from build123d import *
from build123d.topology import SkipClean

# Parameters (mm, degrees)
SKETCH_1_W           = 80
SKETCH_1_H           = 120
SKETCH_1_R           = 1.5
EXTRUDE_2_DEPTH      = 4
SKETCH_4_W           = 4
SKETCH_4_H           = 10
EXTRUDE_4_DEPTH      = 20
EXTRUDE_5_DEPTH      = 15
EXTRUDE_5_DEPTH_BACK = 10
SKETCH_5_W           = 20
SKETCH_5_H           = 4
CUT_EXTRUDE_1_REACH  = 132.959
SKETCH_6_R           = 1.6
CUT_EXTRUDE_START    = -50
CUT_EXTRUDE_3_DEPTH  = 50
EXTRUDE_7_DEPTH      = 15
EXTRUDE_7_DEPTH_BACK = 10
SKETCH_10_W          = 3
SKETCH_10_H          = 3
SKETCH_11_W          = 4
SKETCH_11_H          = 5
EXTRUDE_9_DEPTH      = 15
CUT_EXTRUDE_5_REACH  = 102.708
CUT_EXTRUDE_6_REACH  = 129.241
SKETCH_13_R          = 1.25
SKETCH_13_W          = 22.7
SKETCH_13_H          = 12.5
CUT_EXTRUDE_7_DEPTH  = 114.370984798
SKETCH_15_W          = 6
SKETCH_15_H          = 10
EXTRUDE_10_DEPTH     = 15
CUT_EXTRUDE_8_REACH  = 104.357
EXTRUDE_START        = 3
SKETCH_17_R          = 3
SKETCH_17_R_2        = 1.5
EXTRUDE_11_DEPTH     = 3


with BuildPart() as part:
    # 草图1 → 凸台-拉伸2 (new body)
    with BuildSketch(Plane(origin=(0, 0, 0), x_dir=(1, 0, 0), z_dir=(0, 1, 0))):
        with Locations((1.11138133, -29.732826736)):
            Rectangle(SKETCH_1_W, SKETCH_1_H)
        with Locations(Location((-23.88861867, 20.267173264, 0), (0, 0, 270))):
            Circle(SKETCH_1_R, mode=Mode.SUBTRACT)
        with Locations(Location((26.11138133, 20.267173264, 0), (0, 0, 270))):
            Circle(SKETCH_1_R, mode=Mode.SUBTRACT)
        with Locations(Location((-23.88861867, -64.732826736, 0), (0, 0, 270))):
            Circle(SKETCH_1_R, mode=Mode.SUBTRACT)
        with Locations(Location((26.11138133, -64.732826736, 0), (0, 0, 270))):
            Circle(SKETCH_1_R, mode=Mode.SUBTRACT)
    extrude(amount=EXTRUDE_2_DEPTH)

    # 草图4 → 凸台-拉伸4 (add)
    with BuildSketch(Plane(origin=(0, 4, 0), x_dir=(1, 0, 0), z_dir=(0, 1, 0))):
        Polygon((-38.88861867, -85.732826736), (-38.88861867, -89.732826736), (41.11138133, -89.732826736), (41.11138133, -85.732826736), (26.11138133, -85.732826736), (22.11138133, -85.732826736), (-19.88861867, -85.732826736), (-23.88861867, -85.732826736), align=None)
        with Locations((24.11138133, -80.732826736)):
            Rectangle(SKETCH_4_W, SKETCH_4_H)
        with Locations((-21.88861867, -80.732826736)):
            Rectangle(SKETCH_4_W, SKETCH_4_H)
    extrude(amount=EXTRUDE_4_DEPTH)

    # 草图5 → 凸台-拉伸5 (add, two sides: drawn at the far end of the back side and taken through both)
    with BuildSketch(Plane(origin=(0, 4, 0), x_dir=(1, 0, 0), z_dir=(0, 1, 0)).offset(-EXTRUDE_5_DEPTH_BACK)):
        with Locations((1.11138133, 30.267173264)):
            Rectangle(SKETCH_5_W, SKETCH_5_H)
    extrude(amount=EXTRUDE_5_DEPTH + EXTRUDE_5_DEPTH_BACK)

    # 草图6 → 切除-拉伸1 (cut, up to next)
    with BuildSketch(Plane(origin=(0, 0, -32.267173264), x_dir=(-1, 0, 0), z_dir=(0, 0, -1)), mode=Mode.PRIVATE) as cut_extrude_1_sk1:
        with Locations((2.88861867, 9.096659339)):
            Circle(SKETCH_6_R)
    cut_extrude_1_tool1 = extrude(cut_extrude_1_sk1.sketch, amount=-CUT_EXTRUDE_1_REACH, mode=Mode.PRIVATE) & part.part
    # 草图6 → 切除-拉伸1 (cut, up to next)
    with BuildSketch(Plane(origin=(0, 0, -32.267173264), x_dir=(-1, 0, 0), z_dir=(0, 0, -1)), mode=Mode.PRIVATE) as cut_extrude_1_sk2:
        with Locations((-5.11138133, 9.096659339)):
            Circle(SKETCH_6_R)
    cut_extrude_1_tool2 = extrude(cut_extrude_1_sk2.sketch, amount=-CUT_EXTRUDE_1_REACH, mode=Mode.PRIVATE) & part.part
    add(cut_extrude_1_tool1.solids().sort_by_distance((-2.888619, 9.096659, -32.267173))[0], mode=Mode.SUBTRACT)
    add(cut_extrude_1_tool2.solids().sort_by_distance((5.111381, 9.096659, -32.267173))[0], mode=Mode.SUBTRACT)

    # 草图9 → 切除-拉伸3 (cut)
    with BuildSketch(Plane.ZY.offset(23.88861867).offset(CUT_EXTRUDE_START)):
        Polygon((75.732826736, 24), (75.732826736, 4), (85.732826736, 14), (85.732826736, 24), align=None)
    extrude(amount=CUT_EXTRUDE_3_DEPTH, mode=Mode.SUBTRACT)

    # 草图10 → 凸台-拉伸7 (add, two sides: drawn at the far end of the back side and taken through both)
    with BuildSketch(Plane(origin=(0, 4, 0), x_dir=(1, 0, 0), z_dir=(0, 1, 0)).offset(-EXTRUDE_7_DEPTH_BACK)):
        with Locations((0.730413479, 28.094677972)):
            Rectangle(SKETCH_10_W, SKETCH_10_H)
    extrude(amount=EXTRUDE_7_DEPTH + EXTRUDE_7_DEPTH_BACK)

    # 草图11 → 凸台-拉伸9 (add)
    with BuildSketch(Plane(origin=(0, 4, 0), x_dir=(1, 0, 0), z_dir=(0, 1, 0))):
        Polygon((19.905778303, -55.732826736), (-20.094221697, -55.732826736), (-20.094221697, -59.732826736), (-12.422102113, -59.732826736), (-12.094221697, -59.732826736), (-9.202998314, -59.732826736), (-8.094221697, -59.732826736), (7.905778303, -59.732826736), (11.905778303, -59.732826736), (19.905778303, -59.732826736), align=None)
        Polygon((-9.202998314, -59.732826736), (-12.094221697, -59.732826736), (-12.094221697, -64.732826736), (-8.094221697, -64.732826736), (-8.094221697, -59.732826736), align=None)
        with Locations((9.905778303, -62.232826736)):
            Rectangle(SKETCH_11_W, SKETCH_11_H)
    extrude(amount=EXTRUDE_9_DEPTH)

    # 草图12 → 切除-拉伸5 (cut, up to next)
    with BuildSketch(Plane(origin=(0, 4, 0), x_dir=(1, 0, 0), z_dir=(0, 1, 0)), mode=Mode.PRIVATE) as cut_extrude_5_sk1:
        with BuildLine():
            Line((27.11138133, 8.267173264), (27.11138133, -46.732826736))
            ThreePointArc((27.11138133, -46.732826736), (21.11138133, -52.732826736), (15.11138133, -46.732826736))
            Line((15.11138133, -46.732826736), (15.11138133, 8.267173264))
            ThreePointArc((15.11138133, 8.267173264), (21.11138133, 14.267173264), (27.11138133, 8.267173264))
        make_face()
    cut_extrude_5_tool1 = extrude(cut_extrude_5_sk1.sketch, amount=-CUT_EXTRUDE_5_REACH, mode=Mode.PRIVATE) & part.part
    # 草图12 → 切除-拉伸5 (cut, up to next)
    with BuildSketch(Plane(origin=(0, 4, 0), x_dir=(1, 0, 0), z_dir=(0, 1, 0)), mode=Mode.PRIVATE) as cut_extrude_5_sk2:
        with BuildLine():
            Line((-12.88861867, 8.267173264), (-12.88861867, -46.732826736))
            ThreePointArc((-12.88861867, -46.732826736), (-18.88861867, -52.732826736), (-24.88861867, -46.732826736))
            Line((-24.88861867, -46.732826736), (-24.88861867, 8.267173264))
            ThreePointArc((-24.88861867, 8.267173264), (-18.88861867, 14.267173264), (-12.88861867, 8.267173264))
        make_face()
    cut_extrude_5_tool2 = extrude(cut_extrude_5_sk2.sketch, amount=-CUT_EXTRUDE_5_REACH, mode=Mode.PRIVATE) & part.part
    add(cut_extrude_5_tool1.solids().sort_by_distance((21.111381, 4, 19.232827))[0], mode=Mode.SUBTRACT)
    add(cut_extrude_5_tool2.solids().sort_by_distance((-18.888619, 4, 19.232827))[0], mode=Mode.SUBTRACT)

    # 草图13 → 切除-拉伸6 (cut, up to next)
    with BuildSketch(Plane(origin=(0, 0, 85.732826736), x_dir=(-1, 0, 0), z_dir=(0, 0, -1)), mode=Mode.PRIVATE) as cut_extrude_6_sk1:
        with Locations((-34.86138133, 14.25)):
            Circle(SKETCH_13_R)
    cut_extrude_6_tool1 = extrude(cut_extrude_6_sk1.sketch, amount=-CUT_EXTRUDE_6_REACH, mode=Mode.PRIVATE) & part.part
    # 草图13 → 切除-拉伸6 (cut, up to next)
    with BuildSketch(Plane(origin=(0, 0, 85.732826736), x_dir=(-1, 0, 0), z_dir=(0, 0, -1)), mode=Mode.PRIVATE) as cut_extrude_6_sk2:
        with Locations((-7.36138133, 14.25)):
            Circle(SKETCH_13_R)
    cut_extrude_6_tool2 = extrude(cut_extrude_6_sk2.sketch, amount=-CUT_EXTRUDE_6_REACH, mode=Mode.PRIVATE) & part.part
    # 草图13 → 切除-拉伸6 (cut, up to next)
    with BuildSketch(Plane(origin=(0, 0, 85.732826736), x_dir=(-1, 0, 0), z_dir=(0, 0, -1)), mode=Mode.PRIVATE) as cut_extrude_6_sk3:
        with Locations((5.13861867, 14.25)):
            Circle(SKETCH_13_R)
    cut_extrude_6_tool3 = extrude(cut_extrude_6_sk3.sketch, amount=-CUT_EXTRUDE_6_REACH, mode=Mode.PRIVATE) & part.part
    # 草图13 → 切除-拉伸6 (cut, up to next)
    with BuildSketch(Plane(origin=(0, 0, 85.732826736), x_dir=(-1, 0, 0), z_dir=(0, 0, -1)), mode=Mode.PRIVATE) as cut_extrude_6_sk4:
        with Locations((32.63861867, 14.25)):
            Circle(SKETCH_13_R)
    cut_extrude_6_tool4 = extrude(cut_extrude_6_sk4.sketch, amount=-CUT_EXTRUDE_6_REACH, mode=Mode.PRIVATE) & part.part
    # 草图13 → 切除-拉伸6 (cut, up to next)
    with BuildSketch(Plane(origin=(0, 0, 85.732826736), x_dir=(-1, 0, 0), z_dir=(0, 0, -1)), mode=Mode.PRIVATE) as cut_extrude_6_sk5:
        with Locations((-21.11138133, 14.25)):
            Rectangle(SKETCH_13_W, SKETCH_13_H)
    cut_extrude_6_tool5 = extrude(cut_extrude_6_sk5.sketch, amount=-CUT_EXTRUDE_6_REACH, mode=Mode.PRIVATE) & part.part
    # 草图13 → 切除-拉伸6 (cut, up to next)
    with BuildSketch(Plane(origin=(0, 0, 85.732826736), x_dir=(-1, 0, 0), z_dir=(0, 0, -1)), mode=Mode.PRIVATE) as cut_extrude_6_sk6:
        with Locations((18.88861867, 14.25)):
            Rectangle(SKETCH_13_W, SKETCH_13_H)
    cut_extrude_6_tool6 = extrude(cut_extrude_6_sk6.sketch, amount=-CUT_EXTRUDE_6_REACH, mode=Mode.PRIVATE) & part.part
    add(cut_extrude_6_tool1.solids().sort_by_distance((34.861381, 14.25, 85.732827))[0], mode=Mode.SUBTRACT)
    add(cut_extrude_6_tool2.solids().sort_by_distance((7.361381, 14.25, 85.732827))[0], mode=Mode.SUBTRACT)
    add(cut_extrude_6_tool3.solids().sort_by_distance((-5.138619, 14.25, 85.732827))[0], mode=Mode.SUBTRACT)
    add(cut_extrude_6_tool4.solids().sort_by_distance((-32.638619, 14.25, 85.732827))[0], mode=Mode.SUBTRACT)
    add(cut_extrude_6_tool5.solids().sort_by_distance((21.111381, 14.25, 85.732827))[0], mode=Mode.SUBTRACT)
    add(cut_extrude_6_tool6.solids().sort_by_distance((-18.888619, 14.25, 85.732827))[0], mode=Mode.SUBTRACT)

    # 草图14 → 切除-拉伸7 (cut, through all)
    with BuildSketch(Plane(origin=(26.11138133, 0, 0), x_dir=(0, 0, -1), z_dir=(1, 0, 0))):
        Polygon((-85.732826736, 4), (-75.732826736, 4), (-85.732826736, 14), (-85.732826736, 8), align=None)
    extrude(amount=-CUT_EXTRUDE_7_DEPTH, mode=Mode.SUBTRACT)

    # 草图15 → 凸台-拉伸10 (add)
    with BuildSketch(Plane(origin=(0, 4, 0), x_dir=(1, 0, 0), z_dir=(0, 1, 0))):
        with Locations((1.11138133, -80.732826736)):
            Rectangle(SKETCH_15_W, SKETCH_15_H)
    extrude(amount=EXTRUDE_10_DEPTH)

    # 草图16 → 切除-拉伸8 (cut, up to next)
    with BuildSketch(Plane(origin=(4.11138133, 0, 0), x_dir=(0, 0, -1), z_dir=(1, 0, 0)), mode=Mode.PRIVATE) as cut_extrude_8_sk1:
        Polygon((-85.732826736, 19), (-75.732826736, 4), (-75.732826736, 19), align=None)
    cut_extrude_8_tool1 = extrude(cut_extrude_8_sk1.sketch, amount=-CUT_EXTRUDE_8_REACH, mode=Mode.PRIVATE) & part.part
    add(cut_extrude_8_tool1.solids().sort_by_distance((4.111381, 14, 79.06616))[0], mode=Mode.SUBTRACT)

    # 草图17 → 凸台-拉伸11 (add)
    # profile 1 of 4: a face of its own
    with SkipClean():  # the faces are left unmerged after this step: merging them gives an invalid solid
        with BuildSketch(Plane.XZ.offset(EXTRUDE_START)):
            with Locations(Location((-23.88861867, 64.732826736, 0), (0, 0, 90))):
                Circle(SKETCH_17_R)
            with Locations(Location((-23.88861867, 64.732826736, 0), (0, 0, 270))):
                Circle(SKETCH_17_R_2, mode=Mode.SUBTRACT)
        # profile 2 of 4: a face of its own
        with BuildSketch(Plane.XZ.offset(EXTRUDE_START)):
            with Locations(Location((26.11138133, 64.732826736, 0), (0, 0, 90))):
                Circle(SKETCH_17_R)
            with Locations(Location((26.11138133, 64.732826736, 0), (0, 0, 270))):
                Circle(SKETCH_17_R_2, mode=Mode.SUBTRACT)
        # profile 3 of 4: a face of its own
        with BuildSketch(Plane.XZ.offset(EXTRUDE_START)):
            with Locations(Location((26.11138133, -20.267173264, 0), (0, 0, 90))):
                Circle(SKETCH_17_R)
            with Locations(Location((26.11138133, -20.267173264, 0), (0, 0, 270))):
                Circle(SKETCH_17_R_2, mode=Mode.SUBTRACT)
        # profile 4 of 4: a face of its own
        with BuildSketch(Plane.XZ.offset(EXTRUDE_START)):
            with Locations(Location((-23.88861867, -20.267173264, 0), (0, 0, 90))):
                Circle(SKETCH_17_R)
            with Locations(Location((-23.88861867, -20.267173264, 0), (0, 0, 270))):
                Circle(SKETCH_17_R_2, mode=Mode.SUBTRACT)
        extrude(amount=-EXTRUDE_11_DEPTH)


solid = part.part
Design review of the part built by this model. Coordinates are the model's own, in mm. A direction names the side the tool comes from. Give positions to 0.01 mm unless a question says otherwise; leave off trailing zeros. Write each loop counter-clockwise with the first axis right and the second up, starting at its lowest first coordinate (ties: lowest second). Pieces come first, ordered by that corner, then holes. Notation, with made-up numbers: M 48,0 L 97,0 A24 cw 97,15 Z; hole C 57.5,-35.5 d2. An arc over 180 degrees is marked long. Return JSON: item names as keys, results as strings. Group by question number.
Item 1: Clearance check with flat-ended pins moving along their axes: pin 1 Ø4.5 at (x, z) = (-9.5, 60.5) entering from +Y; pin 2 Ø3 at (x, z) = (-24.5, 15) entering from -Y; pin 3 Ø6.5 at (x, y) = (17, 13) entering from +Z; pin 4 Ø12 at (y, z) = (7.5, -5) entering from +X. State where each tip first meets the part, or that it passes through.
Item 2: Wall thickness on line 1 along Z through (x, y) = (-8.5, 7.5); line 2 along Z through (x, y) = (-6, 5.5); line 3 along Y through (x, z) = (-30, 58): over which ranges is each line inside the solid? List them lowest first.
Item 3: Take a section at A-A (x = 31). Give the boundary of the cut face in (y, z).
Item 4: The part is to be moulded in two halves that separate along X. For faces 6 (the flat face through (1, 11, -26.595)), 7 (the flat face through (-1.889, 10, 82)), 8 (the flat face through (7.906, 11, 62)), say which applies: pulls with the +X half, pulls with the -X half, needs draft (parallel to the pull), parting line crosses it, or undercut.
Item 5: Tool access review of faces 1 (the cylindrical face through (-4.415, 9.577, -30.295)), 2 (the cylindrical face through (25.979, -1.521, 61.736)), 3 (the flat face through (-20.094, 11, 58)), 4 (the flat face through (2, 21, 85.733)), 5 (the cylindrical face through (20.979, 2.028, -14.266)): name each direction out of +Z, -Z, +X, -X, +Y, -Y from which nothing blocks a thin tool from reaching the whole face with its end or side.
Item 6: Take a section at B-B (z = 35.5). Give the boundary of the cut face in (x, y), plus the area to 3 significant figures.
Item 7: Take a section at C-C (y = 14.25). Count the separate pieces of the cut face and the enclosed holes in it, plus the area to 3 significant figures.
Return value:
{
 "1": {"pin 1": "stops at y = 19", "pin 2": "stops at y = 0", "pin 3": "stops at z = 59.73", "pin 4": "stops at x = 41.11"},
 "2": {"line 1": "z = -32.27 to -28.27, 55.73 to 64.73, 85.73 to 89.73", "line 2": "z = -32.27 to -28.27, 55.73 to 59.73, 85.73 to 89.73", "line 3": "y = 0 to 4"},
 "3": {"outline": "M 0,-30.27 L 4,-30.27 L 4,85.73 L 8,85.73 L 8,89.73 L 0,89.73 Z; M 20.5,85.73 L 24,85.73 L 24,89.73 L 20.5,89.73 Z"},
 "4": {"face 6": "needs draft", "face 7": "pulls with the -X half", "face 8": "undercut"},
 "5": {"face 1": "-Z", "face 2": "-Y", "face 3": "-Z, -X, +Y", "face 4": "+Y", "face 5": "+Y, -Y"},
 "6": {"outline": "M -38.89,0 L -24.89,0 L -24.89,4 L -38.89,4 Z; M -12.89,0 L 15.11,0 L 15.11,4 L -12.89,4 Z; M 27.11,0 L 41.11,0 L 41.11,4 L 27.11,4 Z", "area": "224 mm2"},
 "7": {"separate pieces": "9", "enclosed holes": "0", "area": "402 mm2"}
}
